```python
from build123d import *

# Parameters (mm, degrees)
F0_R        = 1.25
F1_DEPTH    = 0.5
F2_R        = 5
F3_T1_DEPTH = 74.0375335511
F3_T3_DEPTH = 9.1893951821
F3_T5_DEPTH = 38.8426126869
F3_T7_DEPTH = 73.4476683762
F4_R        = 100
F5_R        = 5
F6_R        = 2


# Not quite as in the source:
# - a fillet or chamfer that OpenCascade refuses, or shapes differently, is made with other operations: its cross-section is extruded or revolved along the edge and cut away or added


with BuildPart() as f1:
    # F0 (on Front) → F1 (new body)
    with BuildSketch(Plane.XZ):
        with BuildLine():
            Line((-65, 0), (-24, 0))
            Line((-24, 0), (-24, 84))
            Line((-24, 84), (0, 84))
            Line((0, 84), (0, 140))
            Line((0, 140), (-35, 140))
            Line((-35, 140), (-84, 137))
            Line((-84, 137), (-132, 130))
            Line((-132, 130), (-180, 120))
            Line((-180, 120), (-211, 110))
            Line((-211, 110), (-230, 102))
            Line((-230, 102), (-227, 130))
            Line((-227, 130), (-235.2838218212, 130))
            Line((-235.2838218212, 130), (-256, 120))
            Line((-256, 120), (-275, 110))
            Line((-275, 110), (-302, 90))
            Line((-302, 90), (-311, 78))
            Line((-311, 78), (-311, 0))
            Line((-311, 0), (-270, 0))
            Line((-270, 0), (-229, 0))
            Line((-229, 0), (-188, 0))
            Line((-188, 0), (-188, 58.0417635664))
            ThreePointArc((-188, 58.0417635664), (-189.5, 67), (-188, 75.9582364336))
            ThreePointArc((-188, 75.9582364336), (-157.4585244689, 94.1224077102), (-134.5, 67))
            ThreePointArc((-134.5, 67), (-137.8261504927, 53.8898893979), (-147, 43.9511388568))
            Line((-147, 43.9511388568), (-147, 0))
            Line((-147, 0), (-106, 0))
            Line((-106, 0), (-106, 36.0192378865))
            ThreePointArc((-106, 36.0192378865), (-112.1995806787, 83.2268174498), (-65, 76.9666295471))
            ThreePointArc((-65, 76.9666295471), (-62.0172465076, 69.7459666924), (-61, 62))
            ThreePointArc((-61, 62), (-62.0172465076, 54.2540333076), (-65, 47.0333704529))
            Line((-65, 47.0333704529), (-65, 0))
        make_face()
        with Locations((-281, 10)):
            Circle(F0_R, mode=Mode.SUBTRACT)
        with Locations((-240, 10)):
            Circle(F0_R, mode=Mode.SUBTRACT)
        with Locations((-199, 10)):
            Circle(F0_R, mode=Mode.SUBTRACT)
        with Locations((-117, 10)):
            Circle(F0_R, mode=Mode.SUBTRACT)
        with Locations((-35, 10)):
            Circle(F0_R, mode=Mode.SUBTRACT)
        Polygon((-331, 0), (-311, 0), (-311, 78), (-317, 70), (-328, 40), align=None)
        with Locations((-322, 10)):
            Circle(F0_R, mode=Mode.SUBTRACT)
        with BuildLine():
            Line((-188, 0), (-147, 0))
            Line((-147, 0), (-147, 43.9511388568))
            ThreePointArc((-147, 43.9511388568), (-170.9379206853, 40.9930091356), (-188, 58.0417635664))
            Line((-188, 58.0417635664), (-188, 0))
        make_face()
        with Locations((-158, 10)):
            Circle(F0_R, mode=Mode.SUBTRACT)
        with BuildLine():
            Line((-106, 0), (-65, 0))
            Line((-65, 0), (-65, 47.0333704529))
            ThreePointArc((-65, 47.0333704529), (-83.2168271863, 33.0272158578), (-106, 36.0192378865))
            Line((-106, 36.0192378865), (-106, 0))
        make_face()
        with Locations((-76, 10)):
            Circle(F0_R, mode=Mode.SUBTRACT)
    extrude(amount=F1_DEPTH)

    # F2
    f2_edges = [f1.edges().sort_by_distance(p)[0] for p in [
        (-230, -0.25, 102),
    ]]
    fillet(f2_edges, radius=F2_R)

    # F3: fillet of radius 100 on 4 edges, made by hand

    # F3_s2 → F3_t1 (cut)
    with BuildSketch(Plane.XZ.offset(-36.7687667756)):
        with BuildLine():
            ThreePointArc((-308.1754959739, 81.7660053682), (-316.0546249868, 69.4866370062), (-322.0631275625, 56.191470284))
            Line((-322.0631275625, 56.191470284), (-317, 70))
            Line((-317, 70), (-308.1754959739, 81.7660053682))
        make_face()
    extrude(amount=F3_T1_DEPTH, mode=Mode.SUBTRACT)

    # F3_s4 → F3_t3 (cut)
    with BuildSketch(Plane.XZ.offset(-4.3446975911)):
        with BuildLine():
            ThreePointArc((-254.4349231681, 120.7554853112), (-255.9932004856, 119.9865175696), (-257.5378808276, 119.1905890381))
            Line((-257.5378808276, 119.1905890381), (-256, 120))
            Line((-256, 120), (-254.4349231681, 120.7554853112))
        make_face()
    extrude(amount=F3_T3_DEPTH, mode=Mode.SUBTRACT)

    # F3_s6 → F3_t5 (cut)
    with BuildSketch(Plane.XZ.offset(-19.1713063434)):
        with BuildLine():
            ThreePointArc((-268.2139846679, 113.5715870169), (-274.8437916361, 109.7514039115), (-281.1620964472, 105.4354841132))
            Line((-281.1620964472, 105.4354841132), (-275, 110))
            Line((-275, 110), (-268.2139846679, 113.5715870169))
        make_face()
    extrude(amount=F3_T5_DEPTH, mode=Mode.SUBTRACT)

    # F3_s8 → F3_t7 (cut)
    with BuildSketch(Plane.XZ.offset(-36.4738341881)):
        with BuildLine():
            ThreePointArc((-290.2764752677, 98.6840923943), (-301.2536395134, 89.2491836695), (-310.7537202051, 78.3283730598))
            Line((-310.7537202051, 78.3283730598), (-302, 90))
            Line((-302, 90), (-290.2764752677, 98.6840923943))
        make_face()
    extrude(amount=F3_T7_DEPTH, mode=Mode.SUBTRACT)

    # F4
    f4_edges = [f1.edges().sort_by_distance(p)[0] for p in [
        (-328, -0.25, 40),
    ]]
    fillet(f4_edges, radius=F4_R)

    # F5
    f5_edges = [f1.edges().sort_by_distance(p)[0] for p in [
        (-227, -0.25, 130),
    ]]
    fillet(f5_edges, radius=F5_R)

    # F6
    f6_edges = [f1.edges().sort_by_distance(p)[0] for p in [
        (-24, -0.25, 84),
    ]]
    fillet(f6_edges, radius=F6_R)


solid = f1.part
```
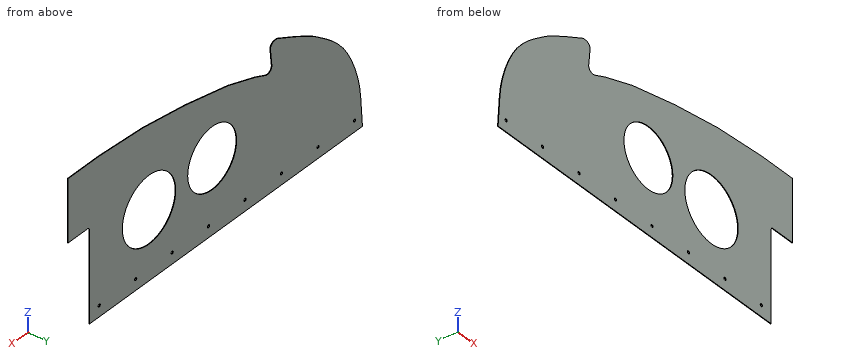
CAD build for the part. Positions are in the model's coordinates, mm. Round coordinates to 2 decimals unless told otherwise and drop trailing zeros. Order: outer loops, then holes, each group sorted by start corner. A loop starts at its lowest first (then second) coordinate and runs counter-clockwise, first axis right, second up. Notation, with made-up numbers: (38.25, 11) - (74.25, 11) arc R30 ccw to (74.25, 43) - close; hole circle Ø9 at (67, -16). An arc over 180 degrees is marked (long way). Answer in a Markdown table with one row per item. Add a question column.
(1) Band-saw the part on A-A on x = -91. List the corners of the cut face in (y, z).
(2) Drop flat-ended pins along their axis: pin 1 Ø1.5 at (x, z) = (-281, 10) entering from +Y; pin 2 Ø3 at (x, z) = (-158, 10) entering from +Y. Give the stop position or say it passes through.
(3) Band-saw the part on B-B on y = -0.4. Count the separate pieces of the cut face and the enclosed holes in it, and give its area (3 significant figures).
(4) Band-saw the part on C-C on x = -140. List the corners of the cut face in (y, z), and give its area (3 significant figures).
(5) Probe L1, parallel to X at y = -0.3, z = 74; L2, parallel to X at y = -0.25, z = 49; L3, parallel to Z at x = -76, y = -0.3. List the from-to ranges inside material, lowest first. Write a range as [from, to].
Data:
| question | item | result |
|---|---|---|
| 1 | outline | (-0.5, 0) - (0, 0) - (0, 32) - (-0.5, 32) - close; (-0.5, 92) - (0, 92) - (0, 135.98) - (-0.5, 135.98) - close |
| 2 | pin 1 | passes through |
| 2 | pin 2 | stops at y = 0 |
| 3 | separate pieces | 1 |
| 3 | enclosed holes | 10 |
| 3 | area | 32,500 mm^2 |
| 4 | outline | (-0.5, 0) - (0, 0) - (0, 50.5) - (-0.5, 50.5) - close; (-0.5, 83.5) - (0, 83.5) - (0, 128.33) - (-0.5, 128.33) - close |
| 4 | area | 47.7 mm^2 |
| 5 | L1 | x = [-313.45, -188.59], [-135.41, -118.5], [-63.5, -24] |
| 5 | L2 | x = [-324.6, -182.79], [-141.21, -118.04], [-63.96, -24] |
| 5 | L3 | z = [0, 8.75], [11.25, 36.02], [87.98, 137.49] |
